```python
from build123d import *

# Parameters (mm, degrees)
SKETCH1_R          = 4
BASE_FLANGE1_DEPTH = 5


# Sheet-metal steps are written as plain solids
with BuildPart() as part:
    # Sketch1 → Base-Flange1 (new body)
    with BuildSketch(Plane.XY):
        with BuildLine():
            Line((-35, 140), (35, 140))
            ThreePointArc((35, 140), (45.606601718, 135.606601718), (50, 125))
            Line((50, 125), (50, -125))
            ThreePointArc((50, -125), (45.606601718, -135.606601718), (35, -140))
            Line((35, -140), (-35, -140))
            ThreePointArc((-35, -140), (-45.606601718, -135.606601718), (-50, -125))
            Line((-50, -125), (-50, 125))
            ThreePointArc((-50, 125), (-45.606601718, 135.606601718), (-35, 140))
        make_face()
        with Locations((0, -114.537631935)):
            Circle(SKETCH1_R, mode=Mode.SUBTRACT)
    extrude(amount=-BASE_FLANGE1_DEPTH)


solid = part.part
```
Work out the finished part from the listing and answer in its coordinate system (mm). Give positions to 0.01 mm unless a question says otherwise; leave off trailing zeros. Loops run counter-clockwise (first coordinate to the right, second up) from the corner with the lowest first, then second, coordinate; pieces in that order, holes last. Notation, with made-up numbers: (-4, 21) -> (27, 21) arc R23 ccw to (27, 45) -> close; hole circle Ø4 at (40, -15.5). An arc over 180 degrees is marked (long way). One line per question, with ' | ' between items. Start each with the question number.
1) Determine the mould class of faces 1 (the face through (1, 2, -5)), 2 (the face through (-0.52, -110.57, -2.46)), 3 (the face through (45.49, 135.72, -2.46)) for opening direction Y: +Y half, -Y half, draft (parallel to the pull), parting line (faces both ways), or undercut.
2) Section A-A, the plane x = 0 is taken. Determine the outline of the cut face in (y, z).
3) Straight lines are drawn through the part: L1, parallel to Y at x = 0, z = -1.9; L2, parallel to X at y = -112, z = -3.75; L3, parallel to Y at x = 45.5, z = -3.55. For each, find the intervals that lie inside material, in ascending order.
Resolved:
1) face 1: draft | face 2: undercut | face 3: +Y half
2) outline: (-140, -5) -> (-118.54, -5) -> (-118.54, 0) -> (-140, 0) -> close; (-110.54, -5) -> (140, -5) -> (140, 0) -> (-110.54, 0) -> close
3) L1: -140 to -118.54, -110.54 to 140 | L2: -50 to -3.09, 3.09 to 50 | L3: -135.71 to 135.71
